The model under review builds one solid part; all positions refer to its coordinate system, in mm. A direction names the side the tool comes from. Round coordinates to 2 decimals unless told otherwise and drop trailing zeros. Loops run counter-clockwise (first coordinate to the right, second up) from the corner with the lowest first, then second, coordinate; pieces in that order, holes last. Notation, with made-up numbers: M -34.5,-23 L 5.5,-23 A23 ccw 5.5,-15 Z; hole C 41.5,18.5 d9. An arc over 180 degrees is marked long. Answer in a Markdown table with one row per item. Add a question column.
from build123d import *

# Parameters (mm, degrees)
SKETCH2_R           = 50
SKETCH2_R_2         = 35
SKETCH2_R_3         = 5.5
BOSS_EXTRUDE1_DEPTH = 10
SKETCH3_R           = 1.5
CUT_EXTRUDE1_DEPTH  = 5


with BuildPart() as part:
    # Sketch2 → Boss-Extrude1 (new body)
    # profile 1 of 11: a face of its own
    with BuildSketch(Plane(origin=(0, 0, 0), x_dir=(1, 0, 0), z_dir=(0, 1, 0))):
        with Locations(Location((0, 0, 0), (0, 0, 270))):
            Circle(SKETCH2_R)
        Circle(SKETCH2_R_2, mode=Mode.SUBTRACT)
    # profile 2 of 11: a face of its own
    with BuildSketch(Plane(origin=(0, 0, 0), x_dir=(1, 0, 0), z_dir=(0, 1, 0))):
        with BuildLine():
            ThreePointArc((-4.763139721, -2.75), (-4.763139721, 2.75), (0, 5.5))
            Line((0, 5.5), (-7.157003146, 9.632097693))
            ThreePointArc((-7.157003146, 9.632097693), (-10.392304845, 6), (-11.920142867, 1.382097693))
            Line((-11.920142867, 1.382097693), (-4.763139721, -2.75))
        make_face()
    # profile 3 of 11: a face of its own
    with BuildSketch(Plane(origin=(0, 0, 0), x_dir=(1, 0, 0), z_dir=(0, 1, 0))):
        with BuildLine():
            Line((-7.157003146, 9.632097693), (0, 5.5))
            Line((0, 5.5), (7.157003146, 9.632097693))
            ThreePointArc((7.157003146, 9.632097693), (0, 12), (-7.157003146, 9.632097693))
        make_face()
    # profile 4 of 11: a face of its own
    with BuildSketch(Plane(origin=(0, 0, 0), x_dir=(1, 0, 0), z_dir=(0, 1, 0))):
        with BuildLine():
            Line((7.157003146, 9.632097693), (0, 5.5))
            ThreePointArc((0, 5.5), (3.889087297, 3.889087297), (5.5, 0))
            ThreePointArc((5.5, 0), (5.312592045, -1.423504748), (4.763139721, -2.75))
            Line((4.763139721, -2.75), (11.920142867, 1.382097693))
            ThreePointArc((11.920142867, 1.382097693), (10.392304845, 6), (7.157003146, 9.632097693))
        make_face()
    # profile 5 of 11: a face of its own
    with BuildSketch(Plane(origin=(0, 0, 0), x_dir=(1, 0, 0), z_dir=(0, 1, 0))):
        with BuildLine():
            ThreePointArc((12, 0), (11.980019082, 0.692201415), (11.920142867, 1.382097693))
            Line((11.920142867, 1.382097693), (4.763139721, -2.75))
            Line((4.763139721, -2.75), (4.763139721, -11.014195386))
            ThreePointArc((4.763139721, -11.014195386), (10.028900155, -6.589473551), (12, 0))
        make_face()
    # profile 6 of 11: a face of its own
    with BuildSketch(Plane(origin=(0, 0, 0), x_dir=(1, 0, 0), z_dir=(0, 1, 0))):
        with BuildLine():
            ThreePointArc((4.763139721, -2.75), (0, -5.5), (-4.763139721, -2.75))
            Line((-4.763139721, -2.75), (-4.763139721, -11.014195386))
            ThreePointArc((-4.763139721, -11.014195386), (0, -12), (4.763139721, -11.014195386))
            Line((4.763139721, -11.014195386), (4.763139721, -2.75))
        make_face()
    # profile 7 of 11: a face of its own
    with BuildSketch(Plane(origin=(0, 0, 0), x_dir=(1, 0, 0), z_dir=(0, 1, 0))):
        with BuildLine():
            Line((-4.763139721, -11.014195386), (-4.763139721, -2.75))
            Line((-4.763139721, -2.75), (-11.920142867, 1.382097693))
            ThreePointArc((-11.920142867, 1.382097693), (-10.392304845, -6), (-4.763139721, -11.014195386))
        make_face()
    # profile 8 of 11: a face of its own
    with BuildSketch(Plane(origin=(0, 0, 0), x_dir=(1, 0, 0), z_dir=(0, 1, 0))):
        Circle(SKETCH2_R_3)
    # profile 9 of 11: a face of its own
    with BuildSketch(Plane(origin=(0, 0, 0), x_dir=(1, 0, 0), z_dir=(0, 1, 0))):
        with BuildLine():
            ThreePointArc((4.763139721, -11.014195386), (0, -12), (-4.763139721, -11.014195386))
            Line((-4.763139721, -11.014195386), (-4.763139721, -34.674378149))
            ThreePointArc((-4.763139721, -34.674378149), (0, -35), (4.763139721, -34.674378149))
            Line((4.763139721, -34.674378149), (4.763139721, -11.014195386))
        make_face()
    # profile 10 of 11: a face of its own
    with BuildSketch(Plane(origin=(0, 0, 0), x_dir=(1, 0, 0), z_dir=(0, 1, 0))):
        with BuildLine():
            ThreePointArc((-11.920142867, 1.382097693), (-10.392304845, 6), (-7.157003146, 9.632097693))
            Line((-7.157003146, 9.632097693), (-27.647322477, 21.462189074))
            ThreePointArc((-27.647322477, 21.462189074), (-30.310889132, 17.5), (-32.410462198, 13.212189074))
            Line((-32.410462198, 13.212189074), (-11.920142867, 1.382097693))
        make_face()
    # profile 11 of 11: a face of its own
    with BuildSketch(Plane(origin=(0, 0, 0), x_dir=(1, 0, 0), z_dir=(0, 1, 0))):
        with BuildLine():
            Line((27.647322477, 21.462189074), (7.157003146, 9.632097693))
            ThreePointArc((7.157003146, 9.632097693), (10.392304845, 6), (11.920142867, 1.382097693))
            Line((11.920142867, 1.382097693), (32.410462198, 13.212189074))
            ThreePointArc((32.410462198, 13.212189074), (30.310889132, 17.5), (27.647322477, 21.462189074))
        make_face()
    extrude(amount=BOSS_EXTRUDE1_DEPTH)

    # Sketch3 → Cut-Extrude1 (cut)
    with BuildSketch(Plane(origin=(0, 10, 0), x_dir=(1, 0, 0), z_dir=(0, 1, 0))):
        with Locations(Location((0, 8, 0), (0, 0, 270))):
            Circle(SKETCH3_R)
        with Locations(Location((8, 0, 0), (0, 0, 270))):
            Circle(SKETCH3_R)
        with Locations(Location((0, -8, 0), (0, 0, 270))):
            Circle(SKETCH3_R)
        with Locations(Location((-8, 0, 0), (0, 0, 270))):
            Circle(SKETCH3_R)
    extrude(amount=-CUT_EXTRUDE1_DEPTH, mode=Mode.SUBTRACT)


solid = part.part
1. Machinability: for faces 1 (the flat face through (-1, 0, -1)), 2 (the cylindrical face through (-10.446, 4.93, 5.907)), 3 (the flat face through (-8, 5, 0)), which of the approach directions +Z, -Z, +X, -X, +Y, -Y give a long, thin tool a straight path to every point of the face, cutting with its end or side? Answer none if there is none.
2. Take a section at D-D, the plane y = 8.5. State the section outline as (x, z) points, and give its area (3 significant figures).
3. For pin 1 Ø2.5 at (x, z) = (8, 0) entering from +Y; pin 2 Ø6 at (x, y) = (-34, 7) entering from -Z; pin 3 Ø1 at (x, y) = (15.5, 8.5) entering from -Z, all flat-tipped, find the tip position at first contact; note any pin that passes through.
4. Mouldability with a two-part tool opening along X and no side actions: class faces 4 (the flat face through (-1, 10, -1)), 5 (the cylindrical face through (15.02, 4.93, 47.69)), 6 (the flat face through (17.546, 4.93, -15.63)) as released by +X, released by -X, zero draft, split by the parting line, or undercut.
5. Take a section at C-C, the plane z = 8. State the section outline as (x, y) points, and give its area (3 significant figures).
6. To check wall thickness, follow probe 1 along Z at (x, y) = (-18.5, 3.25); probe 2 along X at (y, z) = (7.6, -8); probe 3 along X at (y, z) = (8.15, 8). State the ranges of each line that lie inside material, in increasing order.
7. Take a section at A-A, the plane x = 0. State the section outline as (y, z) points.
8. Take a section at B-B, the plane y = 3.5. State the section outline as (x, z) points.
Check sheet entries:
| question | item | result |
|---|---|---|
| 1 | face 1 | +Z, -Z, +X, -X, -Y |
| 1 | face 2 | +Y, -Y |
| 1 | face 3 | +Y |
| 2 | outline | C 0,0 d100; hole M -32.41,-13.21 L -11.92,-1.38 A12 cw -4.76,11.01 L -4.76,34.67 A35 ccw Z; hole M -27.65,-21.46 A35 ccw 27.65,-21.46 L 7.16,-9.63 A12 cw -7.16,-9.63 Z; hole C -8,0 d3; hole C 0,-8 d3; hole C 0,8 d3; hole M 4.76,11.01 A12 cw 11.92,-1.38 L 32.41,-13.21 A35 ccw 4.76,34.67 Z; hole C 8,0 d3 |
| 2 | area | 5,090 mm^2 |
| 3 | pin 1 | stops at y = 5 |
| 3 | pin 2 | stops at z = -39.23 |
| 3 | pin 3 | stops at z = -47.7 |
| 4 | face 4 | zero draft |
| 4 | face 5 | split by the parting line |
| 4 | face 6 | undercut |
| 5 | outline | M -49.36,0 L -34.07,0 L -34.07,10 L -49.36,10 Z; M -8.94,0 L 8.94,0 L 8.94,10 L 1.5,10 L 1.5,5 L -1.5,5 L -1.5,10 L -8.94,10 Z; M 34.07,0 L 49.36,0 L 49.36,10 L 34.07,10 Z |
| 5 | area | 470 mm^2 |
| 6 | probe 1 | z = -46.45 to -29.71, -16.18 to -5.18, 29.71 to 46.45 |
| 6 | probe 2 | x = -49.36 to -34.07, -23.38 to -1.5, 1.5 to 23.38, 34.07 to 49.36 |
| 6 | probe 3 | x = -49.36 to -34.07, -8.94 to -1.5, 1.5 to 8.94, 34.07 to 49.36 |
| 7 | outline | M 0,-50 L 10,-50 L 10,-35 L 0,-35 Z; M 0,-12 L 10,-12 L 10,-9.5 L 5,-9.5 L 5,-6.5 L 10,-6.5 L 10,6.5 L 5,6.5 L 5,9.5 L 10,9.5 L 10,50 L 0,50 Z |
| 8 | outline | C 0,0 d100; hole M -32.41,-13.21 L -11.92,-1.38 A12 cw -4.76,11.01 L -4.76,34.67 A35 ccw Z; hole M -27.65,-21.46 A35 ccw 27.65,-21.46 L 7.16,-9.63 A12 cw -7.16,-9.63 Z; hole M 4.76,11.01 A12 cw 11.92,-1.38 L 32.41,-13.21 A35 ccw 4.76,34.67 Z |
